Job drawing, mm, ordinate dimensions from the low corner. One solid piece. A direction names the side the tool comes from. Coordinates: 2 decimals unless noted, no trailing zeros. Write each loop counter-clockwise with the first axis right and the second up, starting at its lowest first coordinate (ties: lowest second). Pieces come first, ordered by that corner, then holes. Notation, with made-up numbers: (-11, -14) - (3, -14) arc R10 ccw to (3, -1) - close; hole circle Ø10 at (32.25, 82.25). An arc over 180 degrees is marked (long way). Use a Markdown table: item, result.
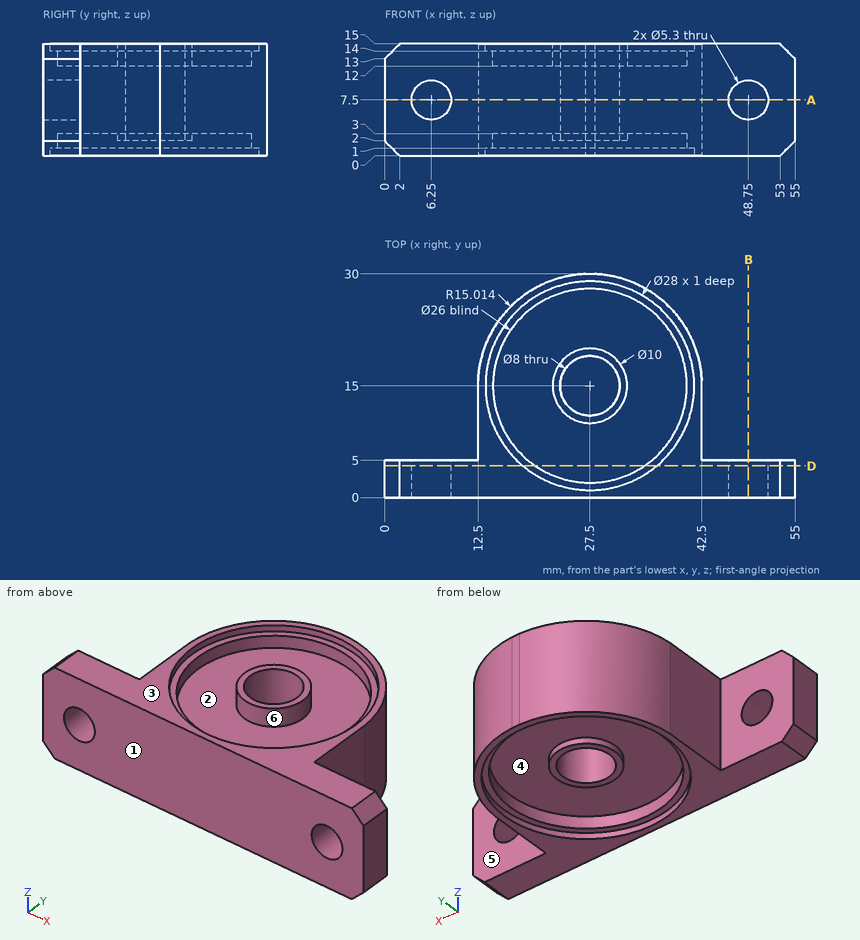
Item 1: Two-plate mould, pull along Y, no slides. Class the marked faces 1, 2 and 3: pulls with the +Y half, pulls with the -Y half, needs draft (parallel to the pull), parting line crosses it, or undercut.
From the geometry:
| item | result |
|---|---|
| face 1 | pulls with the -Y half |
| face 2 | undercut |
| face 3 | needs draft |
Item 2: Drop flat-ended pins along their axis: P1, Ø13, axis at x = 27.5, y = 13, coming from the -Z side; P2, Ø8.5, axis at y = 9.5, z = 5, coming from the +X side; P3, Ø6, axis at y = 23, z = 3.5, coming from the +X side; P4, Ø1, axis at x = 11.5, y = 22, coming from the +Z side. Give the stop position or say it passes through.
From the geometry:
| item | result |
|---|---|
| P1 | z = 2 |
| P2 | x = 42.5 |
| P3 | x = 41.66 |
| P4 | through |
Item 3: Band-saw the part on D-D, the plane y = 4.25. Give the cut face in (x, z).
From the geometry:
| item | result |
|---|---|
| outline | (0, 2) - (2, 0) - (18.53, 0) - (18.53, 1) - (20.19, 1) - (20.19, 3) - (34.81, 3) - (34.81, 1) - (36.47, 1) - (36.47, 0) - (53, 0) - (55, 2) - (55, 13) - (53, 15) - (36.47, 15) - (36.47, 14) - (34.81, 14) - (34.81, 12) - (20.19, 12) - (20.19, 14) - (18.53, 14) - (18.53, 15) - (2, 15) - (0, 13) - close; hole circle Ø5.3 at (6.25, 7.5); hole circle Ø5.3 at (48.75, 7.5) |
Item 4: Band-saw the part on A-A, the plane z = 7.5. Give the cut face in (x, y).
From the geometry:
| item | result |
|---|---|
| outline | (0, 0) - (3.6, 0) - (3.6, 5) - (0, 5) - close; (8.9, 0) - (46.1, 0) - (46.1, 5) - (42.5, 5) - (42.5, 15.65) arc R15.01 ccw to (28.15, 30) - (26.85, 30) arc R15.01 ccw to (12.5, 15.65) - (12.5, 5) - (8.9, 5) - close; (51.4, 0) - (55, 0) - (55, 5) - (51.4, 5) - close; hole circle Ø8 at (27.5, 15) |
Item 5: Band-saw the part on B-B, the plane x = 48.75. Give the cut face in (y, z), then the cut area to 3 significant figures.
From the geometry:
| item | result |
|---|---|
| outline | (0, 0) - (5, 0) - (5, 4.85) - (0, 4.85) - close; (0, 10.15) - (5, 10.15) - (5, 15) - (0, 15) - close |
| area | 48.5 mm^2 |
Item 6: Drill centre lines: probe 1 along Y at (x, z) = (27.5, 10.5); probe 2 along Y at (x, z) = (27.5, 14.65); probe 3 along Z at (x, y) = (49, 3). Where is each one in solid material? Low to high.
From the geometry:
| item | result |
|---|---|
| probe 1 | 0 to 11, 19 to 30 |
| probe 2 | 0 to 1, 10 to 11, 19 to 20, 29 to 30 |
| probe 3 | 0 to 4.86, 10.14 to 15 |
Item 7: Which spindle directions (+Z, -Z, +X, -X, +Y, -Y) get a long thin tool onto all of the face, cutting with end or side? Do the marked faces 4, 5 and 6. Say none if no direction does.
From the geometry:
| item | result |
|---|---|
| face 4 | -Z |
| face 5 | +Z, -Z, +X, +Y |
| face 6 | +Z |
